from build123d import *

# Parameters (mm, degrees)
EXTRUDE_1_DEPTH              = 20
HOLE_WIZARD_M3_1_D           = 2.5
HOLE_WIZARD_M3_1_DEPTH       = 9.5
HOLE_WIZARD_M3_1_TIP         = 0.751075774
HOLE_WIZARD_M4_1_D           = 4.5
HOLE_WIZARD_M4_1_DEPTH       = 9.5
HOLE_WIZARD_M4_1_CBORE_D     = 8
HOLE_WIZARD_M4_1_CBORE_DEPTH = 4.4
HOLE_WIZARD_M4_1_TIP         = 1.351936393


with BuildPart() as part:
    # 草图1 → 凸台-拉伸1 (new body)
    with BuildSketch(Plane.XY):
        Polygon((-6, 13), (-1.75, 13), (-1.75, 34.16), (0.25, 34.16), (0.25, 52.16), (6.25, 52.16), (6.25, 10), (0, 10), (0, 0), (-9, 0), (-9, 11), (-6, 11), align=None)
    extrude(amount=EXTRUDE_1_DEPTH)

    # M3 螺纹孔1
    with Locations(Plane(origin=(6.25, 0, 0), x_dir=(0, 0, -1), z_dir=(1, 0, 0))):
        with Locations((-2.5, 48.66), (-2.5, 37.66), (-5, 31.26), (-15, 31.26), (-17.5, 37.66), (-17.5, 48.66)):
            Hole(HOLE_WIZARD_M3_1_D / 2, depth=HOLE_WIZARD_M3_1_DEPTH)
            with Locations((0, 0, -(HOLE_WIZARD_M3_1_DEPTH + HOLE_WIZARD_M3_1_TIP / 2))):  # 118° drill point
                Cone(0, HOLE_WIZARD_M3_1_D / 2, HOLE_WIZARD_M3_1_TIP, mode=Mode.SUBTRACT)

    # M4 六角凹头螺钉的柱形沉头孔1
    with Locations(Plane.ZY.offset(9)):
        with Locations((5, 4.96), (15, 4.96)):
            CounterBoreHole(HOLE_WIZARD_M4_1_D / 2, HOLE_WIZARD_M4_1_CBORE_D / 2, HOLE_WIZARD_M4_1_CBORE_DEPTH, depth=HOLE_WIZARD_M4_1_DEPTH)
            with Locations((0, 0, -(HOLE_WIZARD_M4_1_DEPTH + HOLE_WIZARD_M4_1_TIP / 2))):  # 118° drill point
                Cone(0, HOLE_WIZARD_M4_1_D / 2, HOLE_WIZARD_M4_1_TIP, mode=Mode.SUBTRACT)


solid = part.part
Could you check a few things on this model? Use its own coordinates, in mm. A direction names the side the tool comes from. Give positions to 0.01 mm unless a question says otherwise; leave off trailing zeros. Order: outer loops, then holes, each group sorted by start corner. A loop starts at its lowest first (then second) coordinate and runs counter-clockwise, first axis right, second up.
Item 1: For faces 5 (the face through (0.25, 43, 10)), 6 (the face through (-7, 5, 11)), 7 (the face through (0, 5, 10)), which set-ups out of +Z, -Z, +X, -X, +Y, -Y let a thin tool reach every point of the face, with its end or its side?
Item 2: I need wall thicknesses on line 1 (Y direction, x = 4.9, z = 17.5); line 2 (Y direction, x = 1.5, z = 5); line 3 (Y direction, x = -7.2, z = 5). Which ranges of each line are inside material? Lowest first, please.
Item 3: If we section it at B-B, the plane z = 5: Write out the boundary of the cut face in (x, y), plus the area to 3 significant figures.
Item 4: If we section it at C-C, the plane x = -5.5: Write out the boundary of the cut face in (y, z), plus the area to 3 significant figures.
Item 5: If we section it at D-D, the plane x = 2.75: Write out the boundary of the cut face in (y, z), plus the area to 3 significant figures.
Item 6: If we section it at A-A, the plane y = 31.26: Write out the boundary of the cut face in (x, z), plus the area to 3 significant figures.
Item 7: If we mould it in two halves opening along Y, with no side actions, what happens to faces 1 (the face through (-6.831, 6.161, 8.815)), 2 (the face through (-4.6, 3, 17)), 3 (the face through (0, 26, 0)), 4 (the face through (3, 52.16, 10))? For each: pulls with the +Y half, pulls with the -Y half, needs draft (parallel to the pull), parting line crosses it, or undercut.
Item 8: I'm going to push flat-ended pins straight in: pin 1 (1.5 mm diameter, centred on x = -7, z = 14.5, fed in from +Y); pin 2 (4 mm diameter, centred on y = 37.66, z = 17.5, fed in from -X); pin 3 (4 mm diameter, centred on x = 3.5, z = 9, fed in from -Y). Where does each tip first touch, or does it pass through?
Values:
1. face 5: +Z, -Z, -X, +Y
1. face 6: -X
1. face 7: +Z, -Z, +X, -Y
2. line 1: y = 10 to 36.41, 38.91 to 47.41, 49.91 to 52.16
2. line 2: y = 10 to 30.01, 32.51 to 52.16
2. line 3: y = 0 to 0.96, 8.96 to 11
3. outline: (-9, 0) - (0, 0) - (0, 2.71) - (-4.6, 2.71) - (-4.6, 0.96) - (-9, 0.96) - close; (-9, 8.96) - (-4.6, 8.96) - (-4.6, 7.21) - (0, 7.21) - (0, 10) - (6.25, 10) - (6.25, 30.01) - (-1.75, 30.01) - (-1.75, 13) - (-6, 13) - (-6, 11) - (-9, 11) - close; (-1.75, 32.51) - (6.25, 32.51) - (6.25, 52.16) - (0.25, 52.16) - (0.25, 34.16) - (-1.75, 34.16) - close
3. area: 331 mm2
4. outline: (0, 0) - (13, 0) - (13, 20) - (0, 20) - close; hole circle Ø8 at (4.96, 5); hole circle Ø8 at (4.96, 15)
4. area: 159 mm2
5. outline: (10, 0) - (52.16, 0) - (52.16, 20) - (10, 20) - close; hole circle Ø2.5 at (31.26, 5); hole circle Ø2.5 at (31.26, 15); hole circle Ø2.5 at (37.66, 2.5); hole circle Ø2.5 at (37.66, 17.5); hole circle Ø2.5 at (48.66, 2.5); hole circle Ø2.5 at (48.66, 17.5)
5. area: 814 mm2
6. outline: (-1.75, 0) - (6.25, 0) - (6.25, 3.75) - (-1.75, 3.75) - close; (-1.75, 6.25) - (6.25, 6.25) - (6.25, 13.75) - (-1.75, 13.75) - close; (-1.75, 16.25) - (6.25, 16.25) - (6.25, 20) - (-1.75, 20) - close
6. area: 120 mm2
7. face 1: undercut
7. face 2: undercut
7. face 3: needs draft
7. face 4: pulls with the +Y half
8. pin 1: stops at y = 11
8. pin 2: stops at x = 0.25
8. pin 3: stops at y = 10
